from build123d import *

# Parameters (mm, degrees)
SKETCH1_R           = 10
SKETCH1_R_2         = 1
BOSS_EXTRUDE1_DEPTH = 2
SKETCH2_R           = 4.5
BOSS_EXTRUDE2_DEPTH = 3.2
SKETCH4_R           = 1.5
CUT_EXTRUDE1_DEPTH  = 2


with BuildPart() as part:
    # Sketch1 → Boss-Extrude1 (new body)
    with BuildSketch(Plane.XY):
        Circle(SKETCH1_R)
        with Locations((0, 7)):
            Circle(SKETCH1_R_2, mode=Mode.SUBTRACT)
        with Locations((-3, 7)):
            Circle(SKETCH1_R_2, mode=Mode.SUBTRACT)
        with Locations((3, 7)):
            Circle(SKETCH1_R_2, mode=Mode.SUBTRACT)
        with Locations((7, 0)):
            Circle(SKETCH1_R_2, mode=Mode.SUBTRACT)
        with Locations((7, -3)):
            Circle(SKETCH1_R_2, mode=Mode.SUBTRACT)
        with Locations((7, 3)):
            Circle(SKETCH1_R_2, mode=Mode.SUBTRACT)
        with Locations((0, -7)):
            Circle(SKETCH1_R_2, mode=Mode.SUBTRACT)
        with Locations((-3, -7)):
            Circle(SKETCH1_R_2, mode=Mode.SUBTRACT)
        with Locations((3, -7)):
            Circle(SKETCH1_R_2, mode=Mode.SUBTRACT)
        with Locations((-7, 0)):
            Circle(SKETCH1_R_2, mode=Mode.SUBTRACT)
        with Locations((-7, 3)):
            Circle(SKETCH1_R_2, mode=Mode.SUBTRACT)
        with Locations((-7, -3)):
            Circle(SKETCH1_R_2, mode=Mode.SUBTRACT)
    extrude(amount=BOSS_EXTRUDE1_DEPTH)

    # Sketch2 → Boss-Extrude2 (add)
    with BuildSketch(Plane.XY.offset(2)):
        Circle(SKETCH2_R)
        Polygon((0.758504156, 2.954178641), (0.975530065, 2.463907688), (1.469348706, 2.672735374), (1.557630919, 2.143895035), (2.087868673, 2.223354314), (2.041860093, 1.689173573), (2.575200173, 1.634271725), (2.397791689, 1.128315123), (2.900722375, 0.942501833), (2.603061214, 0.496560484), (3.043981522, 0.191511085), (2.64477083, -0.166394877), (2.995976115, -0.571513009), (2.520299768, -0.818895035), (2.75972251, -1.298626839), (2.237469003, -1.419941007), (2.35006539, -1.944143169), (1.814049831, -1.931766863), (1.792745019, -2.467501833), (1.276647236, -2.322212702), (1.122779886, -2.835818282), (0.659028201, -2.566745377), (0.382266362, -3.025949839), (0, -2.65), (-0.382266362, -3.025949839), (-0.659028201, -2.566745377), (-1.122779886, -2.835818282), (-1.276647236, -2.322212702), (-1.792745019, -2.467501833), (-1.814049831, -1.931766863), (-2.35006539, -1.944143169), (-2.237469003, -1.419941007), (-2.75972251, -1.298626839), (-2.520299768, -0.818895035), (-2.995976115, -0.571513009), (-2.64477083, -0.166394877), (-3.043981522, 0.191511085), (-2.603061214, 0.496560484), (-2.900722375, 0.942501833), (-2.397791689, 1.128315123), (-2.575200173, 1.634271725), (-2.041860093, 1.689173573), (-2.087868673, 2.223354314), (-1.557630919, 2.143895035), (-1.469348706, 2.672735374), (-0.975530065, 2.463907688), (-0.758504156, 2.954178641), (-0.332133069, 2.629103958), (0, 3.05), (0.332133069, 2.629103958), align=None, mode=Mode.SUBTRACT)
    extrude(amount=BOSS_EXTRUDE2_DEPTH)

    # Sketch4 → Cut-Extrude1 (cut)
    with BuildSketch(Plane.XY.offset(2)):
        Circle(SKETCH4_R)
    extrude(amount=-CUT_EXTRUDE1_DEPTH, mode=Mode.SUBTRACT)


solid = part.part
Input: part model. Units: mm. Frame: model coordinates. A direction names the side the tool comes from. Round coordinates to 2 decimals unless told otherwise and drop trailing zeros. Loops run counter-clockwise (first coordinate to the right, second up) from the corner with the lowest first, then second, coordinate; pieces in that order, holes last. Notation, with made-up numbers: M 36,49.25 L 81,49.25 A26 cw 81,88.25 Z; hole C -12.5,71.5 d7. An arc over 180 degrees is marked long. Answer as CSV lines item,"result". Start each with the question number.
(1) Draft query along X for faces 3 (the cylindrical face through (-3, -6, 1)), 4 (the flat face through (2.1, -4.3, 2)), 5 (the cylindrical face through (-2.17, -9.76, 0.99)). Return one class per face: released by +X, released by -X, zero draft, split by the parting line, or undercut.
(2) First-contact query: pin 1 (1.8 mm diameter, centred on x = 3, y = 7, fed in from +Z); pin 2 (2.5 mm diameter, centred on x = 0, y = -7, fed in from +Z); pin 3 (2 mm diameter, centred on x = 4, z = 4, fed in from -Y); pin 4 (1 mm diameter, centred on x = 1.5, z = 1.5, fed in from +Y). Flat tips, straight axial feed; report the tip coordinate or a pass-through.
(3) Section D-D, the plane y = -3.5. Output: boundary loops of the cut face in (x, z), plus the area to 3 significant figures.
(4) Reachability of faces 1 (the cylindrical face through (-0.59, 4.46, 3.58)), 2 (the cylindrical face through (3, -6, 1)) from +Z, -Z, +X, -X, +Y, -Y: full face, straight path, thin tool, end or side. Return the list, or none.
(5) Line query: line 1 (Y direction, x = 0, z = 1.1); line 2 (Y direction, x = 3, z = 1.15); line 3 (Y direction, x = 7, z = 0.85). Output: solid intervals per line, ascending. Write a range as [from, to].
(6) Section A-A, the plane y = -6.25. Output: boundary loops of the cut face in (x, z), plus the area to 3 significant figures.
(7) Section C-C, the plane x = 6.75. Output: boundary loops of the cut face in (y, z).
(8) Section B-B, the plane z = 0.45. State how many separate pieces and enclosed holes the cut face has, plus the area to 3 significant figures.
Values found:
1,face 3,"undercut"
1,face 4,"zero draft"
1,face 5,"split by the parting line"
2,pin 1,"passes through"
2,pin 2,"stops at z = 2"
2,pin 3,"stops at y = -3.35"
2,pin 4,"stops at y = 9.95"
3,outline,"M -9.37,0 L -7.87,0 L -7.87,2 L -9.37,2 Z; M -6.13,0 L 6.13,0 L 6.13,2 L 2.83,2 L 2.83,5.2 L -2.83,5.2 L -2.83,2 L -6.13,2 Z; M 7.87,0 L 9.37,0 L 9.37,2 L 7.87,2 Z"
3,area,"48.6 mm²"
4,face 1,"+Z"
4,face 2,"+Z, -Z"
5,line 1,"y = [-10, -8], [-6, -1.5], [1.5, 6], [8, 10]"
5,line 2,"y = [-9.54, -8], [-6, 6], [8, 9.54]"
5,line 3,"y = [-7.14, -4], [-2, -1], [1, 2], [4, 7.14]"
6,outline,"M -7.81,0 L -3.66,0 L -3.66,2 L -7.81,2 Z; M -2.34,0 L -0.66,0 L -0.66,2 L -2.34,2 Z; M 0.66,0 L 2.34,0 L 2.34,2 L 0.66,2 Z; M 3.66,0 L 7.81,0 L 7.81,2 L 3.66,2 Z"
6,area,"23.3 mm²"
7,outline,"M -7.38,0 L -3.97,0 L -3.97,2 L -7.38,2 Z; M -2.03,0 L -0.97,0 L -0.97,2 L -2.03,2 Z; M 0.97,0 L 2.03,0 L 2.03,2 L 0.97,2 Z; M 3.97,0 L 7.38,0 L 7.38,2 L 3.97,2 Z"
8,separate pieces,"1"
8,enclosed holes,"13"
8,area,"269 mm²"
